Can you work these out from the model? Positions are in its coordinate system, mm. Face numbers are marked on the shaded views. A direction names the side the tool comes from. Give positions to 0.01 mm unless a question says otherwise; leave off trailing zeros. Order: outer loops, then holes, each group sorted by start corner. A loop starts at its lowest first (then second) coordinate and runs counter-clockwise, first axis right, second up. Notation, with made-up numbers: (-5, 6.5) -> (18, 6.5) arc R18 cw to (18, 12.5) -> close; hole circle Ø6 at (68.5, 41). An arc over 180 degrees is marked (long way). Answer as a JSON object with one key per item and string values.
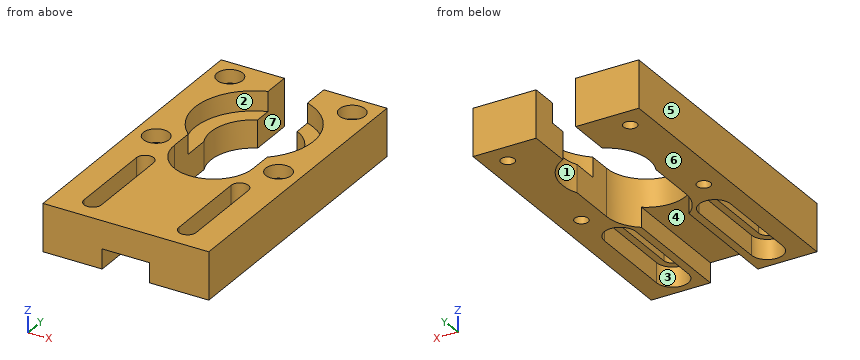
Autodesk Inventor part; units mm, degrees
ref_plane "YZ Plane" through (0, 0, 0) normal (1, 0, 0) x (0, 1, 0)
ref_plane "XZ Plane" through (0, 0, 0) normal (0, 1, 0) x (-1, 0, 0)
ref_plane "XY Plane" through (0, 0, 0) normal (0, 0, 1) x (1, 0, 0)
sketch "Skizze1" plane through (0, 0, 0) normal (0, 0, 1) x (1, 0, 0)
  line L0 (-29.4, 0) -> (29.4, 0)
  line L1 (0, -69) -> (0, 36)
  line L2 (21, -54) -> (-21, -54)
  line L3 (-21, -54) -> (-21, 21)
  line L4 (-21, 21) -> (21, 21)
  line L5 (21, 21) -> (21, -54)
  line L6 (21, -54) -> (-21, 21) construction
  line L7 (-21, -54) -> (21, 21) construction
  circle A0 centre (0, 0) radius 11
  point P0 (0, -16.5)
  dimension "d0" = 42
  dimension "d1" = 75
  dimension "d3" = 22
  dimension "d4" = 21
extrude "Extrusion1" add sketch "Skizze1" along normal blind 12 contours L3 L4 L1 A0 L0 | L0 A0 L1 L2 L3 | L1 L4 L5 L0 A0 | A0 L0 L5 L2 L1
sketch "Skizze2" plane through (0, 0, 12) normal (0, 0, 1) x (1, 0, 0)
  line L0 (21, -54) -> (21, 21)
  line L1 (21, 21) -> (-21, 21)
  line L2 (-21, 21) -> (-21, -54)
  line L3 (-21, -54) -> (21, -54)
  circle A0 centre (0, 0) radius 11
  line L4 (15.5, -15.5) -> (-15.5, -15.5)
  line L5 (-15.5, -15.5) -> (-15.5, 15.5)
  line L6 (-15.5, 15.5) -> (15.5, 15.5)
  line L7 (15.5, 15.5) -> (15.5, -15.5)
  line L8 (15.5, -15.5) -> (-15.5, 15.5) construction
  line L9 (-15.5, -15.5) -> (15.5, 15.5) construction
  dimension "d7" = 31
  dimension "d8" = 31
hole "Bohrung1" at (-15.5, 15.5, 12) at (15.5, 15.5, 12) at (15.5, -15.5, 12) at (-15.5, -15.5, 12) direction (0, 0, -1) diameter 3.4 end through all counterbore diameter 6.5 counterbore depth 3.4
sketch "Skizze3" plane through (0, 0, 0) normal (0, 0, -1) x (-1, 0, 0)
  circle A0 centre (15.5, -15.5) radius 1.7
  circle A1 centre (-15.5, -15.5) radius 1.7
  circle A2 centre (-15.5, 15.5) radius 1.7
  circle A3 centre (15.5, 15.5) radius 1.7
  line L0 (-21, -54) -> (-21, 21)
  line L1 (21, -54) -> (-21, -54)
  line L2 (21, 21) -> (21, -54)
  line L3 (-21, 21) -> (21, 21)
  circle A4 centre (0, 0) radius 11
  line L4 (29.4, 0) -> (-29.4, 0)
  line L5 (0, -69) -> (0, 36)
  line L6 (-12, -48) -> (-12, -26) construction
  line L7 (-8, -48) -> (-8, -26)
  line L8 (-16, -26) -> (-16, -48)
  arc A5 (-16, -48) -> (-8, -48) centre (-12, -48) ccw
  arc A6 (-8, -26) -> (-16, -26) centre (-12, -26) ccw
  line L9 (12, -48) -> (12, -26) construction
  line L10 (16, -48) -> (16, -26)
  line L11 (8, -26) -> (8, -48)
  arc A7 (8, -48) -> (16, -48) centre (12, -48) ccw
  arc A8 (16, -26) -> (8, -26) centre (12, -26) ccw
  point P0 (-12, -37)
  point P1 (12, -37)
  dimension "d16" = 24
  dimension "d17" = 8
  dimension "d18" = 8
  dimension "d19" = 6
  dimension "d20" = 22
extrude "Extrusion2" cut sketch "Skizze3" against normal blind 5 contours A5 L8 A6 L7 | A7 L11 A8 L10
sketch "Skizze4" plane through (0, 0, 0) normal (0, 0, -1) x (-1, 0, 0)
  arc A0 (-8, -26) -> (-16, -26) centre (-12, -26) ccw
  line L0 (-16, -48) -> (-16, -26)
  arc A1 (-16, -48) -> (-8, -48) centre (-12, -48) ccw
  line L1 (-8, -26) -> (-8, -48)
  arc A2 (16, -26) -> (8, -26) centre (12, -26) ccw
  line L2 (8, -48) -> (8, -26)
  arc A3 (8, -48) -> (16, -48) centre (12, -48) ccw
  line L3 (16, -26) -> (16, -48)
  line L4 (12, -48) -> (12, -26) construction
  line L5 (14.2, -48) -> (14.2, -26)
  line L6 (9.8, -26) -> (9.8, -48)
  arc A4 (9.8, -48) -> (14.2, -48) centre (12, -48) ccw
  arc A5 (14.2, -26) -> (9.8, -26) centre (12, -26) ccw
  line L7 (-12, -48) -> (-12, -26) construction
  line L8 (-9.8, -48) -> (-9.8, -26)
  line L9 (-14.2, -26) -> (-14.2, -48)
  arc A6 (-14.2, -48) -> (-9.8, -48) centre (-12, -48) ccw
  arc A7 (-9.8, -26) -> (-14.2, -26) centre (-12, -26) ccw
  point P0 (0, 0)
  point P1 (12, -37)
  point P2 (-12, -37)
  dimension "d23" = 4.4
  dimension "d24" = 4.4
extrude "Extrusion3" cut sketch "Skizze4" against normal through all contours A4 L6 A5 L5 | A6 L9 A7 L8
sketch "Skizze5" plane through (0, 0, 12) normal (0, 0, 1) x (1, 0, 0)
  line L0 (-9.8, -26) -> (-9.8, -48)
  arc A0 (-14.2, -48) -> (-9.8, -48) centre (-12, -48) ccw
  line L1 (-14.2, -48) -> (-14.2, -26)
  arc A1 (-9.8, -26) -> (-14.2, -26) centre (-12, -26) ccw
  line L2 (14.2, -26) -> (14.2, -48)
  arc A2 (9.8, -48) -> (14.2, -48) centre (12, -48) ccw
  line L3 (9.8, -48) -> (9.8, -26)
  arc A3 (14.2, -26) -> (9.8, -26) centre (12, -26) ccw
  circle A4 centre (-15.5, -15.5) radius 3.25
  circle A5 centre (15.5, -15.5) radius 3.25
  circle A6 centre (15.5, 15.5) radius 3.25
  circle A7 centre (-15.5, 15.5) radius 3.25
  line L4 (21, -54) -> (21, 21)
  line L5 (21, 21) -> (-21, 21)
  line L6 (-21, 21) -> (-21, -54)
  line L7 (-21, -54) -> (21, -54)
  circle A8 centre (0, 0) radius 11
  circle A9 centre (0, 0) radius 15
  dimension "d27" = 30
extrude "Extrusion4" cut sketch "Skizze5" against normal blind 5 contours A9
sketch "Skizze6" plane through (0, 0, 12) normal (0, 0, 1) x (1, 0, 0)
  circle A0 centre (0, 0) radius 15
  line L0 (-9.8, -26) -> (-9.8, -48)
  arc A1 (-14.2, -48) -> (-9.8, -48) centre (-12, -48) ccw
  line L1 (-14.2, -48) -> (-14.2, -26)
  arc A2 (-9.8, -26) -> (-14.2, -26) centre (-12, -26) ccw
  line L2 (14.2, -26) -> (14.2, -48)
  arc A3 (9.8, -48) -> (14.2, -48) centre (12, -48) ccw
  line L3 (9.8, -48) -> (9.8, -26)
  arc A4 (14.2, -26) -> (9.8, -26) centre (12, -26) ccw
  circle A5 centre (-15.5, -15.5) radius 3.25
  circle A6 centre (15.5, -15.5) radius 3.25
  circle A7 centre (15.5, 15.5) radius 3.25
  circle A8 centre (-15.5, 15.5) radius 3.25
  line L4 (21, -54) -> (21, 21)
  line L5 (21, 21) -> (-21, 21)
  line L6 (-21, 21) -> (-21, -54)
  line L7 (-21, -54) -> (21, -54)
  line L8 (-29.4, 0) -> (29.4, 0)
  line L9 (0, -69) -> (0, 36)
  line L10 (-5, 8) -> (5, 8)
  line L11 (5, 8) -> (5, 26)
  line L12 (5, 26) -> (-5, 26)
  line L13 (-5, 26) -> (-5, 8)
  line L14 (-5, 8) -> (5, 26) construction
  line L15 (5, 8) -> (-5, 26) construction
  point P0 (0, 17)
  dimension "d30" = 18
  dimension "d31" = 10
  dimension "d32" = 8
extrude "Extrusion5" cut sketch "Skizze6" against normal through all contours L11 L10 L9 A0 | A0 L9 L5 L11 | L9 L10 L13 A0 | A0 L13 L5 L9 | L5 L9 L12 L11 | L5 L13 L12 L9
sketch "Skizze7" plane through (0, 0, 12) normal (0, 0, 1) x (1, 0, 0)
  line L0 (5, 14.1421) -> (5, 9.798)
  arc A0 (-5, 9.798) -> (5, 9.798) centre (0, 0) ccw
  line L1 (-5, 9.798) -> (-5, 14.1421)
  arc A1 (-5, 14.1421) -> (5, 14.1421) centre (0, 0) ccw
  line L2 (-29.4, 0) -> (29.4, 0)
  line L3 (0, -69) -> (0, 36)
  line L4 (0, 0) -> (0, -17) construction
  line L5 (-10, 0) -> (-10, -17)
  line L6 (10, -17) -> (10, 0)
  arc A2 (10, 0) -> (-10, 0) centre (0, 0) ccw
  arc A3 (-10, -17) -> (10, -17) centre (0, -17) ccw
  point P0 (0, -8.5)
  dimension "d35" = 20
  dimension "d36" = 17
extrude "Extrusion6" cut sketch "Skizze7" against normal through all contours L6 A3 L3 A1 | A1 L3 A0 L6 | A0 L3 L2 L6 | L2 L3 A2 | L3 A3 L5 A1 | A1 L5 A0 L3 | A0 L5 L2 L3 | L2 A2 L3
sketch "Skizze8" plane through (0, 0, 0) normal (0, 0, -1) x (-1, 0, 0)
  line L0 (-5, 9.798) -> (-5, 21)
  line L1 (-21, 21) -> (-5, 21)
  line L2 (-21, -54) -> (-21, 21)
  line L3 (21, -54) -> (-21, -54)
  line L4 (21, 21) -> (21, -54)
  line L5 (5, 21) -> (21, 21)
  line L6 (5, 21) -> (5, 9.798)
  arc A0 (-5, 9.798) -> (-10, -4.5826) centre (0, 0) ccw
  circle A1 centre (15.5, 15.5) radius 1.7
  circle A2 centre (-15.5, 15.5) radius 1.7
  circle A3 centre (-15.5, -15.5) radius 1.7
  circle A4 centre (15.5, -15.5) radius 1.7
  line L7 (-16, -48) -> (-16, -26)
  arc A5 (-8, -26) -> (-16, -26) centre (-12, -26) ccw
  line L8 (-8, -26) -> (-8, -48)
  arc A6 (-16, -48) -> (-8, -48) centre (-12, -48) ccw
  line L9 (8, -48) -> (8, -26)
  arc A7 (16, -26) -> (8, -26) centre (12, -26) ccw
  line L10 (16, -26) -> (16, -48)
  arc A8 (8, -48) -> (16, -48) centre (12, -48) ccw
  line L11 (29.4, 0) -> (-29.4, 0)
  line L12 (0, -69) -> (0, 36)
  line L13 (10, -4.5826) -> (10, -17)
  arc A9 (-10, -17) -> (10, -17) centre (0, -17) ccw
  line L14 (-10, -17) -> (-10, -4.5826)
  arc A10 (10, -4.5826) -> (5, 9.798) centre (0, 0) ccw
  line L15 (0, 0) -> (0, -60) construction
  line L16 (-6, 0) -> (-6, -60)
  line L17 (6, -60) -> (6, 0)
  arc A11 (6, 0) -> (-6, 0) centre (0, 0) ccw
  arc A12 (-6, -60) -> (6, -60) centre (0, -60) ccw
  point P0 (0, -30)
  point P1 (11, 0)
  point P2 (21, 0)
  point P3 (-21, 0)
  point P4 (-11, 0)
  point P5 (-6, -25)
  point P6 (6, -25)
  point P7 (0, -66)
  point P8 (0, -54)
  point P9 (-6, -54)
  point P10 (0, 6)
  point P11 (0, -27)
  point P12 (6, -54)
  dimension "d39" = 12
  dimension "d40" = 60
extrude "Extrusion7" cut sketch "Skizze8" against normal blind 5 contours A11 L12 L11 | L11 L12 A9 L16 | L12 A11 L11 | L11 L17 A9 L12 | A9 L12 L3 L16 | A9 L17 L3 L12 | L3 L12 A12 L16 | L3 L17 A12 L12
equation "\"d18\" = d17"
equation "\"d24\" = d23"
properties part number "24_0497_008"
1. If we section it at D-D on x = 9: Please give me the cut outline in (y, z).
Worked answers:
{"outline": "(-54, 0) -> (-50.65, 0) -> (-50.65, 5) -> (-23.35, 5) -> (-23.35, 0) -> (-21.36, 0) -> (-21.36, 12) -> (-54, 12) -> close; (6.32, 0) -> (21, 0) -> (21, 12) -> (12, 12) -> (12, 7) -> (6.32, 7) -> close"}
2. For the marked faces 1, 2, 3 and 4, which set-ups out of +Z, -Z, +X, -X, +Y, -Y let a thin tool reach every point of the face, with its end or its side?
Worked answers:
{"face 1": "+Z, -Z", "face 2": "+Z", "face 3": "-Z", "face 4": "-Z, -Y"}
3. If we section it at C-C on y = 15.5: Please give me the cut outline in (x, z), then the cut area to 3 significant figures.
Worked answers:
{"outline": "(-21, 0) -> (-17.2, 0) -> (-17.2, 8.6) -> (-18.75, 8.6) -> (-18.75, 12) -> (-21, 12) -> close; (-13.8, 0) -> (-5, 0) -> (-5, 12) -> (-12.25, 12) -> (-12.25, 8.6) -> (-13.8, 8.6) -> close; (5, 0) -> (13.8, 0) -> (13.8, 8.6) -> (12.25, 8.6) -> (12.25, 12) -> (5, 12) -> close; (17.2, 0) -> (21, 0) -> (21, 12) -> (18.75, 12) -> (18.75, 8.6) -> (17.2, 8.6) -> close", "area": "281 mm²"}
4. If we section it at B-B on z = 6: Please give me the cut outline in (x, y), then the cut area to 3 significant figures.
Worked answers:
{"outline": "(-21, -54) -> (21, -54) -> (21, 21) -> (5, 21) -> (5, 9.8) arc R11 cw to (10, -4.58) -> (10, -17) arc R10 cw to (-10, -17) -> (-10, -4.58) arc R11 cw to (-5, 9.8) -> (-5, 21) -> (-21, 21) -> close; hole circle Ø3.4 at (-15.5, -15.5); hole circle Ø3.4 at (-15.5, 15.5); hole (-14.2, -48) arc R2.2 ccw to (-9.8, -48) -> (-9.8, -26) arc R2.2 ccw to (-14.2, -26) -> close; hole (9.8, -48) arc R2.2 ccw to (14.2, -48) -> (14.2, -26) arc R2.2 ccw to (9.8, -26) -> close; hole circle Ø3.4 at (15.5, -15.5); hole circle Ø3.4 at (15.5, 15.5)", "area": "2,090 mm²"}
5. Will these pins go through, and if not, where does the flat tip stop? pin 1 Ø2 at (x, y) = (15.5, -15.5) entering from -Z; pin 2 Ø3 at (x, y) = (11.5, 7) entering from +Z; pin 3 Ø1.5 at (x, z) = (-2, 11) entering from +Y; pin 4 Ø6 at (x, y) = (15.5, 15.5) entering from +Z.
Worked answers:
{"pin 1": "through", "pin 2": "z = 7", "pin 3": "y = -26.61", "pin 4": "z = 8.6"}
6. If we mould it in two halves opening along X, with no side actions, what happens to the marked faces 5, 6 and 7? For each: +X half, -X half, draft (parallel to the pull), parting line (faces both ways), or undercut.
Worked answers:
{"face 5": "-X half", "face 6": "draft", "face 7": "undercut"}
7. If we section it at A-A on z = 2.25: Please give me the cut outline in (x, y), then the cut area to 3 significant figures.
Worked answers:
{"outline": "(-21, -54) -> (-6, -54) -> (-6, -25) arc R10 cw to (-10, -17) -> (-10, -4.58) arc R11 cw to (-5, 9.8) -> (-5, 21) -> (-21, 21) -> close; (5, 9.8) arc R11 cw to (10, -4.58) -> (10, -17) arc R10 cw to (6, -25) -> (6, -54) -> (21, -54) -> (21, 21) -> (5, 21) -> close; hole circle Ø3.4 at (-15.5, -15.5); hole circle Ø3.4 at (-15.5, 15.5); hole (-16, -48) arc R4 ccw to (-8, -48) -> (-8, -26) arc R4 ccw to (-16, -26) -> close; hole (8, -48) arc R4 ccw to (16, -48) -> (16, -26) arc R4 ccw to (8, -26) -> close; hole circle Ø3.4 at (15.5, -15.5); hole circle Ø3.4 at (15.5, 15.5)", "area": "1,530 mm²"}
8. Please list where these lines run through material, in increasing order: L1, parallel to X at y = -15.5, z = 10.9; L2, parallel to Y at x = -15.5, z = 5.25; L3, parallel to X at y = -33.5, z = 10.
Worked answers:
{"L1": "-21 to -18.75, -12.25 to -10, 10 to 12.25, 18.75 to 21", "L2": "-54 to -17.2, -13.8 to 13.8, 17.2 to 21", "L3": "-21 to -14.2, -9.8 to 9.8, 14.2 to 21"}
